Autodesk Fusion 360 part; units mm, degrees
sketch "Sketch1" plane through (0, 0, 0) normal (0, 1, 0) x (1, 0, 0)
  line L0 (49, 21) -> (-49, 21)
  line L1 (-49, 21) -> (-49, -21)
  line L2 (-49, -21) -> (49, -21)
  line L3 (49, -21) -> (49, 21)
  line L4 (49, 21) -> (-49, -21) construction
  line L5 (-49, 21) -> (49, -21) construction
  circle A0 centre (25, 0) radius 6
  circle A1 centre (-25, 0) radius 6
  dimension "d1" = 98
  dimension "d2" = 42
  dimension "d3" = 12
  dimension "d4" = 12
  dimension "d5" = 24
  dimension "d6" = 21
  dimension "d8" = 21
  dimension "d16" = 50
extrude "Extrude1" add sketch "Sketch1" along normal blind 20
sketch "Sketch2" plane through (0, 0, 21) normal (0, 0, 1) x (1, 0, 0)
  line L0 (-49, 0) -> (49, 0)
  line L1 (49, 0) -> (49, 20)
  line L2 (49, 20) -> (-49, 20)
  line L3 (-49, 20) -> (-49, 0)
  line L4 (-35, 0) -> (35, 0)
  line L5 (35, 0) -> (35, 9)
  line L6 (35, 9) -> (-35, 9)
  line L7 (-35, 9) -> (-35, 0)
  dimension "d11" = 70
  dimension "d12" = 9
  dimension "d13" = 14
extrude "Extrude2" cut sketch "Sketch2" against normal blind 42 contours L0 L4 L5 L6 L7
sketch "Sketch3" plane through (0, 20, 0) normal (0, 1, 0) x (-1, 0, 0)
  circle A0 centre (25, 0) radius 6
  circle A1 centre (-25, 0) radius 6
  line L0 (-49, 21) -> (-49, -21)
  line L1 (-49, -21) -> (49, -21)
  line L2 (49, -21) -> (49, 21)
  line L3 (49, 21) -> (-49, 21)
  line L4 (-7, -21) -> (7, -21)
  line L5 (7, -21) -> (7, 21)
  line L6 (7, 21) -> (-7, 21)
  line L7 (-7, 21) -> (-7, -21)
  line L8 (-7, -21) -> (7, 21) construction
  line L9 (7, -21) -> (-7, 21) construction
  dimension "d17" = 14
  dimension "d18" = 42
extrude "Extrude3" add sketch "Sketch3" along normal blind 42 contours L1 L3 L4 L5 L6 L7
sketch "Sketch4" plane through (7, 0, 0) normal (1, 0, 0) x (0, 0, -1)
  line L0 (-21, 20) -> (21, 20)
  line L1 (21, 20) -> (21, 62)
  line L2 (21, 62) -> (-21, 62)
  line L3 (-21, 62) -> (-21, 20)
  circle A0 centre (0, 41) radius 10
  arc A1 (21, 41) -> (-21, 41) centre (0, 41) ccw
  dimension "d21" = 42
  dimension "d22" = 21
extrude "Extrude4" cut sketch "Sketch4" against normal blind 14 contours L2 L3 A1 | L1 L2 A1 | A0
fillet "Fillet1" radius 5 2 edges at (49, 20, 0) (-49, 20, 0)
fillet "Fillet2" radius 5 2 edges at (7, 20, 0) (-7, 20, 0)
Can you work these out from the model? Positions are in its coordinate system, mm. A direction names the side the tool comes from. Give positions to 0.01 mm unless a question says otherwise; leave off trailing zeros. Order: outer loops, then holes, each group sorted by start corner. A loop starts at its lowest first (then second) coordinate and runs counter-clockwise, first axis right, second up. Notation, with made-up numbers: M 88.25,-38 L 136.25,-38 A23 ccw 136.25,0 Z; hole C 63.25,0 d5. An arc over 180 degrees is marked long. One line per item, written item: value.
Item 1: If we section it at C-C on x = 3.5: Write out the boundary of the cut face in (y, z).
Verdict:
outline: M 9,-21 L 41,-21 A21 ccw 41,21 L 9,21 Z; hole C 41,0 d20
Item 2: For faces 1 (the face through (-7, 51.5, -0.3)), 2 (the face through (31.3, 20, -0.3)), 3 (the face through (-35, 5, 0)), 4 (the face through (49, 7, 0)), which set-ups out of +Z, -Z, +X, -X, +Y, -Y let a thin tool reach every point of the face, with its end or its side?
Verdict:
face 1: +Z, -Z, -X, +Y
face 2: +Z, -Z, +X, +Y
face 3: +Z, -Z, -Y
face 4: +Z, -Z, +X, +Y, -Y
Item 3: If we section it at D-D on z = -17: Write out the boundary of the cut face in (x, y).
Verdict:
outline: M -49,0 L -35,0 L -35,9 L 35,9 L 35,0 L 49,0 L 49,15 A5 ccw 44,20 L 12,20 A5 cw 7,25 L 7,53.33 L -7,53.33 L -7,25 A5 cw -12,20 L -44,20 A5 ccw -49,15 Z
Item 4: If we section it at B-B on z = 0: Write out the boundary of the cut face in (x, y), and give its area (3 significant figures).
Verdict:
outline: M -49,0 L -35,0 L -35,9 L -31,9 L -31,20 L -44,20 A5 ccw -49,15 Z; M -19,9 L 19,9 L 19,20 L 12,20 A5 cw 7,25 L 7,31 L -7,31 L -7,25 A5 cw -12,20 L -19,20 Z; M -7,51 L 7,51 L 7,62 L -7,62 Z; M 31,9 L 35,9 L 35,0 L 49,0 L 49,15 A5 ccw 44,20 L 31,20 Z
area: 1,370 mm2
Item 5: Please list where these lines run through material, in increasing order: line 1 (X direction, y = 13.75, z = 0); line 2 (Y direction, x = 3, z = 0); line 3 (Z direction, x = -25, y = 12).
Verdict:
line 1: -49 to -31, -19 to 19, 31 to 49
line 2: 9 to 31, 51 to 62
line 3: -21 to -6, 6 to 21
Item 6: For pin 1 (11 mm diameter, centred on y = 38, z = -5, fed in from +X); pin 2 (19 mm diameter, centred on x = 25, z = 0, fed in from +Y); pin 3 (8 mm diameter, centred on x = 1.5, y = 49, fed in from -Z), each with a flat end and sliding along its axis, tell me the tip position at first contact or that it passes through.
Verdict:
pin 1: x = 7
pin 2: y = 20
pin 3: z = -20.62
Item 7: If we section it at A-A on x = 25: Write out the boundary of the cut face in (y, z), and give its area (3 significant figures).
Verdict:
outline: M 9,-21 L 20,-21 L 20,-6 L 9,-6 Z; M 9,6 L 20,6 L 20,21 L 9,21 Z
area: 330 mm2
Item 8: If we mould it in two halves opening along Z, with no side actions, what happens to faces 5 (the face through (0, 13, -21)), 6 (the face through (20.24, 14.42, -3.65)), 7 (the face through (35, 4, 0))? For each: pulls with the +Z half, pulls with the -Z half, needs draft (parallel to the pull), parting line crosses it, or undercut.
Verdict:
face 5: pulls with the -Z half
face 6: undercut
face 7: needs draft
